Drawing for the job (mm, zero at the part's lowest x, y, z). A direction names the side the tool comes from. Give positions to 0.01 mm unless a question says otherwise; leave off trailing zeros. Order: outer loops, then holes, each group sorted by start corner. A loop starts at its lowest first (then second) coordinate and runs counter-clockwise, first axis right, second up. Notation, with made-up numbers: (-38.75, 23) - (16.25, 23) arc R12 ccw to (16.25, 33) - close; hole circle Ø5 at (-38, 80.5). An arc over 180 degrees is marked (long way). Write each question's results on one line, items separated by ' | '. Start each with the question number.
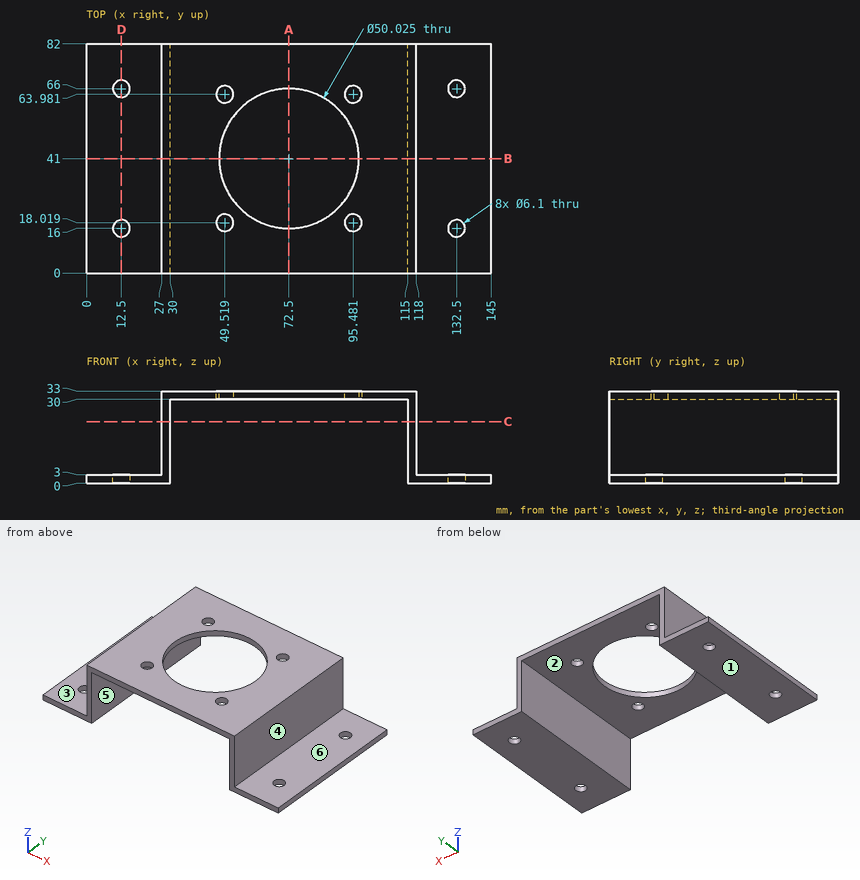
Item 1: Probe line 1 along X through (y, z) = (61, 20); line 2 along X through (y, z) = (61.5, 32.5); line 3 along Y through (x, z) = (72.5, 30.7). List the from-to ranges inside material, lowest first. Write a range as from..to.
Item 2: Cut at A-A, the plane x = 72.5. List the corners of the cut face in (y, z), then the cut area to 3 significant figures.
Item 3: Cut at C-C, the plane z = 22. List the corners of the cut face in (x, y).
Item 4: Flat gauge pins, fed straight in: pin 1 Ø21.5 at (x, y) = (135.5, 46.5) entering from +Z; pin 2 Ø3.5 at (x, y) = (49.519, 18.019) entering from +Z; pin 3 Ø9 at (y, z) = (21.5, 21.5) entering from -X; pin 4 Ø4 at (x, y) = (74, 67) entering from -Z. Where does each tip first touch, or does it go through?
Item 5: Cut at B-B, the plane y = 41. List the corners of the cut face in (x, z).
Item 6: Cut at D-D, the plane x = 12.5. List the corners of the cut face in (y, z), then the cut area to 3 significant figures.
Item 7: Which spindle directions (+Z, -Z, +X, -X, +Y, -Y) get a long thin tool onto all of the face, cutting with end or side? Do the marked faces 1, 2 and 3. Say none if no direction does.
Item 8: Two-plate mould, pull along X, no slides. Class the marked faces 4, 5 and 6: +X half, -X half, draft (parallel to the pull), parting line (faces both ways), or undercut.
Values found:
1) line 1: x = 27..30, 115..118 | line 2: x = 27..47.74, 51.29..58.17, 86.83..93.71, 97.26..118 | line 3: y = 0..15.99, 66.01..82
2) outline: (0, 30) - (15.99, 30) - (15.99, 33) - (0, 33) - close; (66.01, 30) - (82, 30) - (82, 33) - (66.01, 33) - close | area: 95.9 mm2
3) outline: (27, 0) - (30, 0) - (30, 82) - (27, 82) - close; (115, 0) - (118, 0) - (118, 82) - (115, 82) - close
4) pin 1: stops at z = 3 | pin 2: passes through | pin 3: stops at x = 27 | pin 4: stops at z = 30
5) outline: (0, 0) - (30, 0) - (30, 30) - (47.49, 30) - (47.49, 33) - (27, 33) - (27, 3) - (0, 3) - close; (97.51, 30) - (115, 30) - (115, 0) - (145, 0) - (145, 3) - (118, 3) - (118, 33) - (97.51, 33) - close
6) outline: (0, 0) - (12.95, 0) - (12.95, 3) - (0, 3) - close; (19.05, 0) - (62.95, 0) - (62.95, 3) - (19.05, 3) - close; (69.05, 0) - (82, 0) - (82, 3) - (69.05, 3) - close | area: 209 mm2
7) face 1: -Z, +X, -X, +Y, -Y | face 2: -Z, +Y, -Y | face 3: +Z, -X, +Y, -Y
8) face 4: +X half | face 5: undercut | face 6: draft
